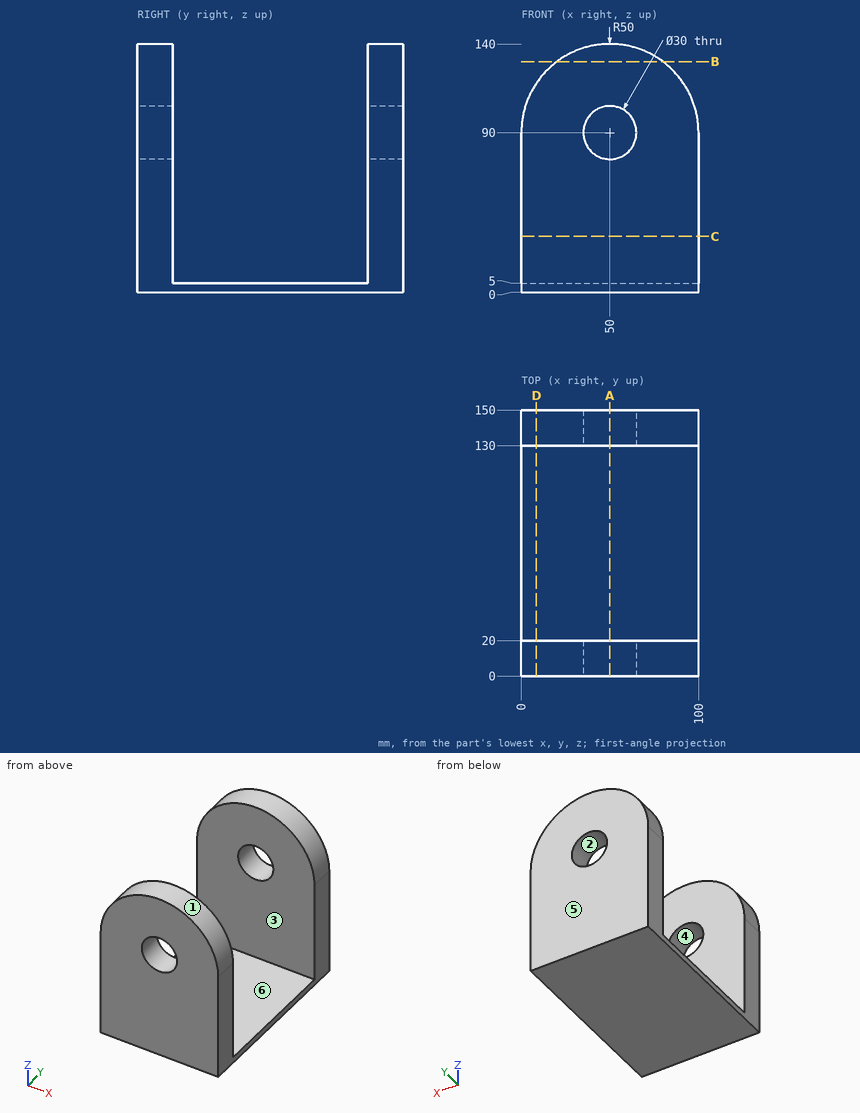
Geometry check sheet. Reference: drawing and pictorial views, mm from the part's lowest x, y, z. A direction names the side the tool comes from. Round coordinates to 2 decimals unless told otherwise and drop trailing zeros. Write each loop counter-clockwise with the first axis right and the second up, starting at its lowest first coordinate (ties: lowest second). Pieces come first, ordered by that corner, then holes. Notation, with made-up numbers: (-22.5, 1.5) -> (-12.5, 1.5) arc R13 ccw to (-12.5, 9.5) -> close; hole circle Ø2 at (59, 60). An arc over 180 degrees is marked (long way). One line per question, with ' | ' between items. Start each with the question number.
1. Sectioned sample at D-D, the plane x = 8.5. Record the cut outline in (y, z), then the cut area to 3 significant figures.
2. Release check for a two-part mould opening along Z. For the marked faces 1, 2, 3 and 4 record: +Z half, -Z half, draft (parallel to the pull), parting line (faces both ways), or undercut.
3. Sectioned sample at C-C, the plane z = 31.5. Record the cut outline in (x, y).
4. Set-up check for the marked faces 5 and 6: record each of +Z, -Z, +X, -X, +Y, -Y from which the full face is reachable in a straight line by a thin tool's end or side.
5. Sectioned sample at B-B, the plane z = 130. Record the cut outline in (x, y).
6. Sectioned sample at A-A, the plane x = 50. Record the cut outline in (y, z), then the cut area to 3 significant figures.
7. Scan lines: line 1 along Y through (x, z) = (20.5, 79); line 2 along Z through (x, y) = (50, 8.5); line 3 along X through (y, z) = (144, 96). Record each from-to range of solid material in increasing order. Write a range as from..to.
Taken from the geometry:
1) outline: (0, 0) -> (150, 0) -> (150, 117.89) -> (130, 117.89) -> (130, 5) -> (20, 5) -> (20, 117.89) -> (0, 117.89) -> close | area: 5,270 mm^2
2) face 1: +Z half | face 2: undercut | face 3: draft | face 4: undercut
3) outline: (0, 0) -> (100, 0) -> (100, 20) -> (0, 20) -> close; (0, 130) -> (100, 130) -> (100, 150) -> (0, 150) -> close
4) face 5: +Z, -Z, +X, -X, +Y | face 6: +Z, +X, -X
5) outline: (20, 0) -> (80, 0) -> (80, 20) -> (20, 20) -> close; (20, 130) -> (80, 130) -> (80, 150) -> (20, 150) -> close
6) outline: (0, 0) -> (150, 0) -> (150, 75) -> (130, 75) -> (130, 5) -> (20, 5) -> (20, 75) -> (0, 75) -> close; (0, 105) -> (20, 105) -> (20, 140) -> (0, 140) -> close; (130, 105) -> (150, 105) -> (150, 140) -> (130, 140) -> close | area: 4,950 mm^2
7) line 1: y = 0..20, 130..150 | line 2: z = 0..75, 105..140 | line 3: x = 0.36..36.25, 63.75..99.64
